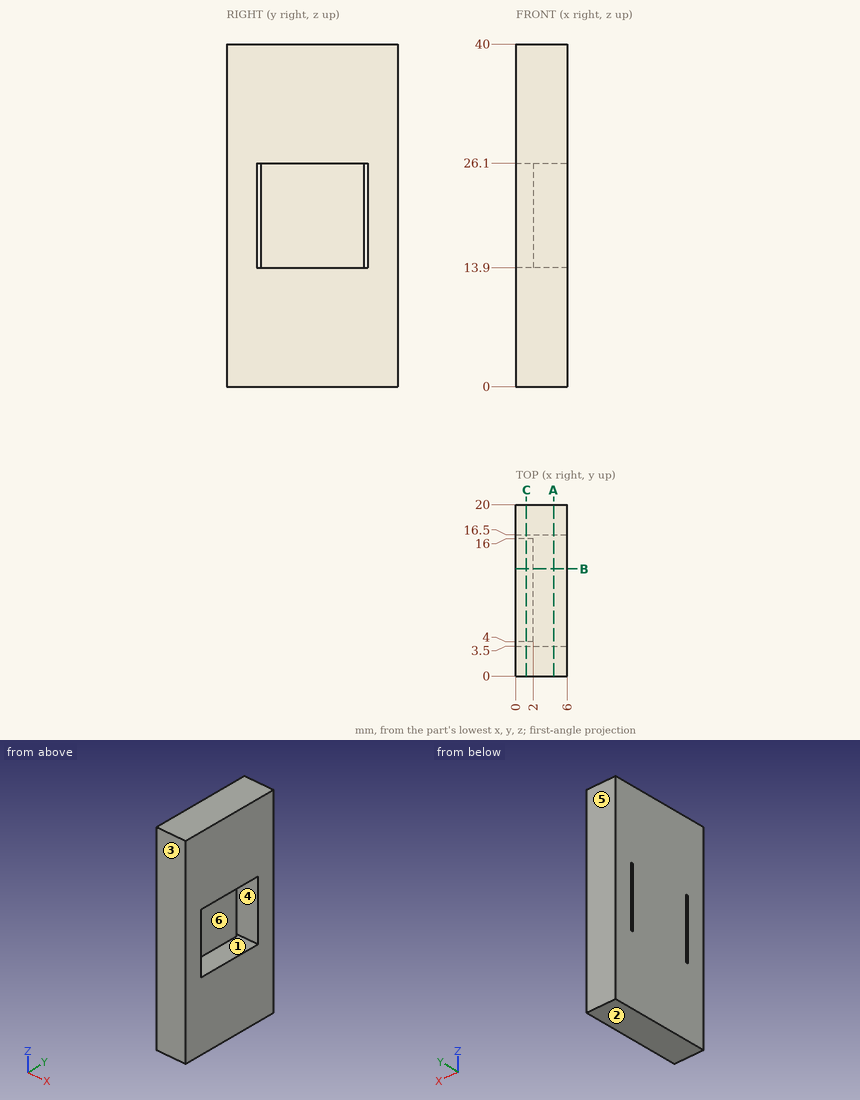
Source: three-view drawing plus pictorial views. Frame: mm from the lowest corner of the part. A direction names the side the tool comes from. Give positions to 0.01 mm unless a question says otherwise; leave off trailing zeros. Write each loop counter-clockwise with the first axis right and the second up, starting at its lowest first coordinate (ties: lowest second). Pieces come first, ordered by that corner, then holes.
(1) Cut plane C-C, the plane x = 1.2. Return loops of the section in (y, z).
(2) Access query for the marked faces 4, 5 and 6. Directions: +Z, -Z, +X, -X, +Y, -Y. A direction counts if a zero-diameter tool reaches every point of the face in a straight line with its end or side. Return the directions, or none.
(3) Cut plane B-B, the plane y = 12.5. Return loops of the section in (x, z).
(4) Ray query, line 1 (Y direction, x = 0.5, z = 25.5); line 2 (Z direction, x = 3.5, y = 9.75); line 3 (Y direction, x = 5.65, z = 14). Return the intervals inside material, ascending.
(5) Mould query, pull axis Z, two halves, no side actions, for the marked faces 1, 2 and 3. Classes: released by +Z, released by -Z, zero draft, split by the parting line, or undercut.
(6) Cut plane A-A, the plane x = 4.4. Return loops of the section in (y, z).
(7) First-contact query: P1, Ø1.8, axis at x = 3, z = 20, coming from the -Y side; P2, Ø6, axis at y = 11.5, z = 20, coming from the +X side. Flat tips, straight axial feed; report the tip coordinate or a pass-through.
Values follow:
1. outline: (0, 0) - (20, 0) - (20, 40) - (0, 40) - close; hole (3.5, 13.9) - (4, 13.9) - (4, 26.1) - (3.5, 26.1) - close; hole (16, 13.9) - (16.5, 13.9) - (16.5, 26.1) - (16, 26.1) - close
2. face 4: +X, -X
2. face 5: +Z, -Z, +X, -X, +Y
2. face 6: +X
3. outline: (0, 0) - (6, 0) - (6, 13.9) - (2, 13.9) - (2, 26.1) - (6, 26.1) - (6, 40) - (0, 40) - close
4. line 1: y = 0 to 3.5, 4 to 16, 16.5 to 20
4. line 2: z = 0 to 13.9, 26.1 to 40
4. line 3: y = 0 to 3.5, 16.5 to 20
5. face 1: undercut
5. face 2: released by -Z
5. face 3: zero draft
6. outline: (0, 0) - (20, 0) - (20, 40) - (0, 40) - close; hole (3.5, 13.9) - (16.5, 13.9) - (16.5, 26.1) - (3.5, 26.1) - close
7. P1: stops at y = 0
7. P2: stops at x = 2
